```python
from build123d import *

# Parameters (mm, degrees)
BODY_DEPTH   = 8.2
SKETCH2_R    = 1.8
SCREWS_DEPTH = 6
SKETCH3_W    = 4
SKETCH3_H    = 4
WIRE_R_DEPTH = 8
SKETCH4_W    = 4
SKETCH4_H    = 4
WIRE_L_DEPTH = 8


with BuildPart() as part:
    # Sketch1 → Body (new body)
    with BuildSketch(Plane(origin=(0, 0, 0), x_dir=(1, 0, 0), z_dir=(0, 1, 0))):
        Polygon((-25, 0), (25, 0), (25, -20), (18, -20), (18, -32), (8, -32), (8, -42), (-8, -42), (-8, -32), (-18, -32), (-18, -20), (-25, -20), align=None)
    extrude(amount=BODY_DEPTH)

    # Sketch2 → Screws (cut)
    with BuildSketch(Plane.XY.offset(20)):
        with Locations((-21.5, 4.1)):
            Circle(SKETCH2_R)
        with Locations((21.5, 4.1)):
            Circle(SKETCH2_R)
    extrude(amount=-SCREWS_DEPTH, mode=Mode.SUBTRACT)

    # Sketch3 → Wire_R (cut)
    with BuildSketch(Plane(origin=(25, 0, 0), x_dir=(0, 0, -1), z_dir=(1, 0, 0))):
        with Locations((-10, 4.1)):
            Rectangle(SKETCH3_W, SKETCH3_H)
    extrude(amount=-WIRE_R_DEPTH, mode=Mode.SUBTRACT)

    # Sketch4 → Wire_L (cut)
    with BuildSketch(Plane(origin=(-25, 0, 0), x_dir=(0, 0, -1), z_dir=(1, 0, 0))):
        with Locations((-10, 4.1)):
            Rectangle(SKETCH4_W, SKETCH4_H)
    extrude(amount=WIRE_L_DEPTH, mode=Mode.SUBTRACT)


solid = part.part
```
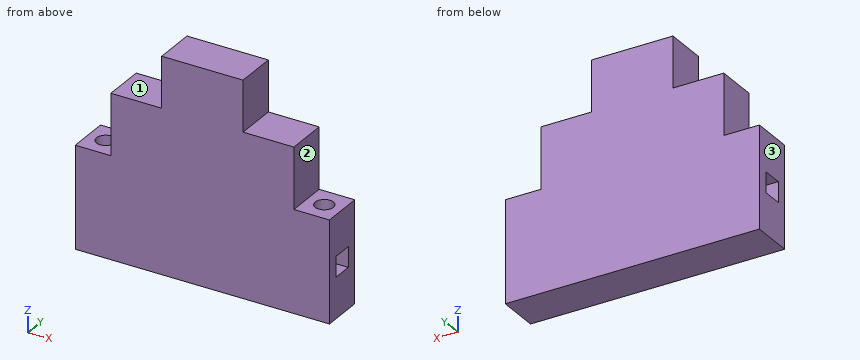
Check sheet for the modelled part. Datum: model origin and axes. Units: mm. Face numbers are marked on the shaded views. A direction names the side the tool comes from. Coordinates: 2 decimals unless noted, no trailing zeros. Write each loop counter-clockwise with the first axis right and the second up, starting at its lowest first coordinate (ties: lowest second). Pieces come first, ordered by that corner, then holes. Notation, with made-up numbers: (29, 1) - (60, 1) arc R15 cw to (60, 22) - close; hole circle Ø1 at (46.5, 74). An arc over 180 degrees is marked (long way). One line per question, with ' | ' between items.
Item 1: Sectioned sample at B-B on y = 7. Record the boundary of the cut face in (x, z).
Determined:
outline: (-25, 0) - (25, 0) - (25, 20) - (18, 20) - (18, 32) - (8, 32) - (8, 42) - (-8, 42) - (-8, 32) - (-18, 32) - (-18, 20) - (-25, 20) - close
Item 2: Access from +Z, -Z, +X, -X, +Y, -Y to the whole of each face (thin tool, end or side, straight path). Record for the marked faces 1, 2 and 3.
Determined:
face 1: +Z, -X, +Y, -Y | face 2: +Z, +X, +Y, -Y | face 3: +Z, -Z, -X, +Y, -Y
Item 3: Sectioned sample at C-C on x = -21.5. Record the boundary of the cut face in (y, z), plus the area to 3 significant figures.
Determined:
outline: (0, 0) - (8.2, 0) - (8.2, 20) - (5.9, 20) - (5.9, 14) - (2.3, 14) - (2.3, 20) - (0, 20) - close; hole (2.1, 8) - (6.1, 8) - (6.1, 12) - (2.1, 12) - close | area: 126 mm2
Item 4: Sectioned sample at D-D on z = 25. Record the boundary of the cut face in (x, y).
Determined:
outline: (-18, 0) - (18, 0) - (18, 8.2) - (-18, 8.2) - close
Item 5: Thickness scan on line 1 (Z direction, x = 23, y = 2.75); line 2 (Y direction, x = 21.5, z = 16.2); line 3 (Z direction, x = 9, y = 7.25). Record the ranges inside material, lowest first. Write a range as [from, to].
Determined:
line 1: z = [0, 8], [12, 20] | line 2: y = [0, 2.3], [5.9, 8.2] | line 3: z = [0, 32]
Item 6: Gauge pin test, flat ends, axial feed: P1, Ø1, axis at y = 1.5, z = 37, coming from the +X side; P2, Ø4, axis at x = 21, y = 3.5, coming from the +Z side; P3, Ø2, axis at x = 21.5, y = 3.5, coming from the +Z side. Record the tip position at first contact, or that the pin passes through.
Determined:
P1: stops at x = 8 | P2: stops at z = 20 | P3: stops at z = 14
Item 7: Sectioned sample at A-A on x = 20.5. Record the boundary of the cut face in (y, z), plus the area to 3 significant figures.
Determined:
outline: (0, 0) - (8.2, 0) - (8.2, 20) - (5.6, 20) - (5.6, 14) - (2.6, 14) - (2.6, 20) - (0, 20) - close; hole (2.1, 8) - (6.1, 8) - (6.1, 12) - (2.1, 12) - close | area: 130 mm2
